Design review of the part built by this model. Coordinates are the model's own, in mm. Face numbers are marked on the shaded views. A direction names the side the tool comes from. Round coordinates to 2 decimals unless told otherwise and drop trailing zeros. Order: outer loops, then holes, each group sorted by start corner. A loop starts at its lowest first (then second) coordinate and runs counter-clockwise, first axis right, second up. Notation, with made-up numbers: M 1.25,-40 L 29.25,-40 A26 cw 29.25,-3 Z; hole C -6,64 d4. An arc over 180 degrees is marked long. Use a Markdown table: item, result. Add a question column.
(1) Take a section at D-D (x = -7.5). Write out the cut boundary in (y, z).
(2) For pin 1 (3 mm diameter, centred on x = -6, y = -1.5, fed in from +Z); pin 2 (2 mm diameter, centred on y = -4, z = 6, fed in from -X), all flat-tipped, find the tip position at first contact; note any pin that passes through.
(3) Take a section at C-C (z = 13). Write out the cut boundary in (x, y).
(4) Machinability: for the marked faces 1, 2 and 3, which of the approach directions +Z, -Z, +X, -X, +Y, -Y give a long, thin tool a straight path to every point of the face, cutting with its end or side? Answer none if there is none.
(5) To check wall thickness, follow probe 1 along Z at (x, y) = (-2.75, -1.8); probe 2 along Z at (x, y) = (-4.25, -2.85); probe 3 along X at (y, z) = (-4.6, -5). State the ranges of each line that lie inside material, in increasing order. Write a range as from..to.
(6) Take a section at B-B (y = -3). Write out the cut boundary in (x, z).
(7) Take a section at A-A (x = 0). Write out the cut boundary in (y, z).
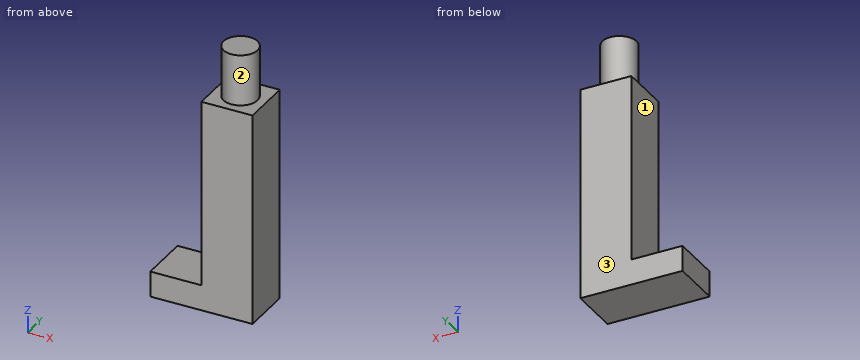
```python
from build123d import *

# Parameters (mm, degrees)
F1_DEPTH = 6
F2_R     = 2
F3_DEPTH = 6


with BuildPart() as f1:
    # F0 (on Front) → F1 (new body)
    with BuildSketch(Plane.XZ):
        Polygon((3, 12.5), (-3, 12.5), (-3, -9.5), (-9, -9.5), (-9, -12.5), (-3, -12.5), (3, -12.5), align=None)
    extrude(amount=F1_DEPTH)

    # F2 (on face) → F3 (join)
    with BuildSketch(Plane.XY.offset(12.5)):
        with Locations((0, -3)):
            Circle(F2_R)
    extrude(amount=F3_DEPTH)


solid = f1.part
```
Verdict:
| question | item | result |
|---|---|---|
| 1 | outline | M -6,-12.5 L 0,-12.5 L 0,-9.5 L -6,-9.5 Z |
| 2 | pin 1 | stops at z = -9.5 |
| 2 | pin 2 | stops at x = -3 |
| 3 | outline | C 0,-3 d4 |
| 4 | face 1 | +Z, -X, +Y, -Y |
| 4 | face 2 | +Z |
| 4 | face 3 | +Z, -Z, +X, -X, +Y |
| 5 | probe 1 | z = -12.5..12.5 |
| 5 | probe 2 | z = -12.5..-9.5 |
| 5 | probe 3 | x = -3..3 |
| 6 | outline | M -9,-12.5 L 3,-12.5 L 3,12.5 L 2,12.5 L 2,18.5 L -2,18.5 L -2,12.5 L -3,12.5 L -3,-9.5 L -9,-9.5 Z |
| 7 | outline | M -6,-12.5 L 0,-12.5 L 0,12.5 L -1,12.5 L -1,18.5 L -5,18.5 L -5,12.5 L -6,12.5 Z |
